Model file for the job. Use its own axes, mm. Round coordinates to 2 decimals unless told otherwise and drop trailing zeros. Write each loop counter-clockwise with the first axis right and the second up, starting at its lowest first coordinate (ties: lowest second). Pieces come first, ordered by that corner, then holes. Notation, with made-up numbers: (49.5, 83) - (68.5, 83) arc R9 ccw to (68.5, 89) - close; hole circle Ø11 at (87.25, 54.25). An arc over 180 degrees is marked (long way). One line per item, written item: value.
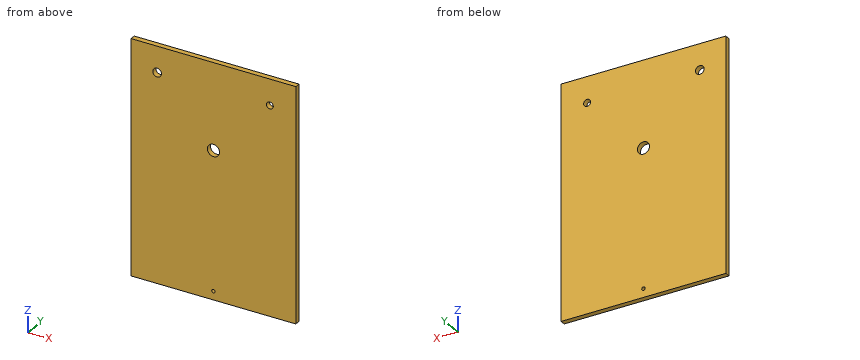
Autodesk Inventor part; units mm, degrees
ref_plane "YZ Plane" through (0, 0, 0) normal (1, 0, 0) x (0, 1, 0)
ref_plane "XZ Plane" through (0, 0, 0) normal (0, 1, 0) x (-1, 0, 0)
ref_plane "XY Plane" through (0, 0, 0) normal (0, 0, 1) x (1, 0, 0)
sketch "Boceto1" plane through (0, 0, 0) normal (0, 1, 0) x (-1, 0, 0)
  line L0 (0, 0) -> (-105, 0)
  line L1 (-105, 0) -> (-105, -140)
  line L2 (-105, -140) -> (0, -140)
  line L3 (0, -140) -> (0, 0)
  dimension "d0" = 105
  dimension "d1" = 140
extrude "Extrusión1" add sketch "Boceto1" along normal blind 3
sketch "Boceto2" plane through (0, 3, 0) normal (0, 1, 0) x (1, 0, 0)
  circle A0 centre (85, 15) radius 2
  circle A1 centre (20, 15) radius 2.5
  circle A2 centre (52.5, 50) radius 3.5
  line L0 (0, 0) -> (105, 0)
  line L1 (0, 140) -> (0, 0)
  line L2 (105, 0) -> (105, 140)
  line L3 (52.5, 50) -> (52.5, -7.4445)
  dimension "d4" = 4
  dimension "d5" = 5
  dimension "d6" = 7
  dimension "d7" = 15
  dimension "d8" = 15
  dimension "d9" = 50
  dimension "d10" = 52.5
  dimension "d11" = 105
  dimension "d14" = 85
  dimension "d15" = 85
extrude "Extrusión2" cut sketch "Boceto2" against normal blind 3
sketch "Boceto3" plane through (0, 3, 0) normal (0, 1, 0) x (1, 0, 0)
  circle A0 centre (20, 15) radius 2.5
  circle A1 centre (85, 15) radius 2
  circle A2 centre (52.5, 50) radius 3.5
  line L0 (0, 0) -> (105, 0)
  line L1 (105, 0) -> (105, 140)
  line L2 (105, 140) -> (0, 140)
  line L3 (0, 140) -> (0, 0)
  circle A3 centre (52.5, 130) radius 1
  dimension "d18" = 2
  dimension "d19" = 0
  dimension "d20" = 10
extrude "Extrusión3" cut sketch "Boceto3" against normal blind 3 contours A3
sketch "Boceto4" plane through (105, 0, -140) normal (0, 0, -1) x (-1, 0, 0)
  line L0 (0, 0) -> (105, 0)
  line L1 (105, 0) -> (105, 3)
  line L2 (0, 3) -> (105, 3)
  line L3 (0, 0) -> (0, 3)
extrude "Extrusión4" cut sketch "Boceto4" against normal blind 5
sketch "Boceto5" plane through (0, 3, 0) normal (0, 1, 0) x (1, 0, 0)
  line L0 (105, 135) -> (0, 135)
  line L1 (0, 135) -> (0, 0)
  line L2 (0, 0) -> (105, 0)
  line L3 (105, 0) -> (105, 135)
  circle A0 centre (52.5, 50) radius 3.5
  circle A1 centre (85, 15) radius 2
  circle A2 centre (20, 15) radius 2.5
  circle A3 centre (52.5, 130) radius 1
  line L4 (105, 135) -> (0, 135)
  line L5 (102.5, 0) -> (2.5, 0)
  line L6 (2.5, 0) -> (2.5, 135)
  line L7 (2.5, 135) -> (102.5, 135)
  line L8 (102.5, 135) -> (102.5, 0)
  line L9 (102.5, 0) -> (2.5, 135) construction
  line L10 (2.5, 0) -> (102.5, 135) construction
  point P0 (52.5, 67.5)
  dimension "d25" = 100
extrude "Extrusión5" cut sketch "Boceto5" against normal blind 3 contours L3 L2 L8 L0 | L6 L2 L1 L0
sketch "Boceto6" plane through (0, 0, 0) normal (0, -1, 0) x (1, 0, 0)
  line L0 (102.5, -135) -> (102.5, 0)
  line L1 (2.5, 0) -> (102.5, 0)
  line L2 (2.5, 0) -> (2.5, -135)
  line L3 (2.5, -135) -> (102.5, -135)
  circle A0 centre (52.5, -130) radius 1
  circle A1 centre (20, -15) radius 2.5
  circle A2 centre (85, -15) radius 2
  circle A3 centre (52.5, -50) radius 3.5
  line L4 (2.5, 0) -> (102.5, 0)
  line L5 (100, -135) -> (5, -135)
  line L6 (5, -135) -> (5, 0)
  line L7 (5, 0) -> (100, 0)
  line L8 (100, 0) -> (100, -135)
  line L9 (100, -135) -> (5, 0) construction
  line L10 (5, -135) -> (100, 0) construction
  point P0 (0, 0)
  point P1 (52.5, -67.5)
  dimension "d28" = 95
extrude "Extrusión6" cut sketch "Boceto6" against normal blind 3 contours L3 L8 L1 L0 | L3 L2 L1 L6
equation "\"d10\" = 0.5 * d11"
properties part number "trasera"
1. Band-saw the part on A-A on x = 20. Write the cut outline in (y, z), plus the area to 3 significant figures.
Report:
outline: (0, -135) - (3, -135) - (3, -17.5) - (0, -17.5) - close; (0, -12.5) - (3, -12.5) - (3, 0) - (0, 0) - close
area: 390 mm²
2. Band-saw the part on C-C on z = -50. Write the cut outline in (x, y), plus the area to 3 significant figures.
Report:
outline: (5, 0) - (49, 0) - (49, 3) - (5, 3) - close; (56, 0) - (100, 0) - (100, 3) - (56, 3) - close
area: 264 mm²
3. Band-saw the part on B-B on z = -15. Write the cut outline in (x, y), plus the area to 3 significant figures.
Report:
outline: (5, 0) - (17.5, 0) - (17.5, 3) - (5, 3) - close; (22.5, 0) - (83, 0) - (83, 3) - (22.5, 3) - close; (87, 0) - (100, 0) - (100, 3) - (87, 3) - close
area: 258 mm²
4. Wall check: probe 1 along Z at (x, y) = (52.5, 2.35); probe 2 along Z at (x, y) = (20, 0.9); probe 3 along X at (y, z) = (1.65, -130). Give the ranges that are in metal, low to high. Write a range as [from, to].
Report:
probe 1: [-135, -131], [-129, -53.5], [-46.5, 0]
probe 2: [-135, -17.5], [-12.5, 0]
probe 3: [5, 51.5], [53.5, 100]
5. Drop a flat-ended pin along its axis: pin 1 (2 mm diameter, centred on x = 21, z = -23, fed in from -Y). Give the stop position or say it passes through.
Report:
pin 1: y = 0
